```python
from build123d import *

# Parameters (mm, degrees)
F1_DEPTH = 25.4
F2_R     = 4.7625
F3_DEPTH = 12.7


with BuildPart() as f1:
    # F0 (on Right) → F1 (new body, symmetric)
    with BuildSketch(Plane.YZ):
        Polygon((787.4, 9.525), (0, 9.525), (-82.55, 9.525), (-82.55, 0), (-142.875, 0), (-133.35, -9.525), (-33.290768, -9.525), (838.2, -9.525), (838.2, 0), (787.4, 0), align=None)
    extrude(amount=F1_DEPTH, both=True)

    # F2 (on Top) → F3 (cut, symmetric)
    with BuildSketch(Plane.XY):
        with Locations((0, 812.8)):
            Circle(F2_R)
        with Locations((0, 447.675)):
            Circle(F2_R)
    extrude(amount=F3_DEPTH, both=True, mode=Mode.SUBTRACT)


solid = f1.part
```
Design review of the part built by this model. Coordinates are the model's own, in mm. A direction names the side the tool comes from. Give positions to 0.01 mm unless a question says otherwise; leave off trailing zeros. Use a Markdown table: item, result. Add a question column.
(1) Clearance check with flat-ended pins moving along their axes: P1, Ø4, axis at x = 16.5, z = 5, coming from the -Y side; P2, Ø11, axis at x = 0, y = 812.8, coming from the +Z side; P3, Ø11, axis at x = 0, y = 447.675, coming from the -Z side (3 decimals); P4, Ø1, axis at x = 20, z = -6, coming from the -Y side (3 decimals). State where each tip first meets the part, or that it passes through.
(2) Machinability: for faces 1 (the face through (0.4, 807.5, 0)), 2 (the face through (0, -112, 0)), 3 (the face through (-25.4, 341, 0)), which of the approach directions +Z, -Z, +X, -X, +Y, -Y give a long, thin tool a straight path to every point of the face, cutting with its end or side? Answer none if there is none.
(3) Wall thickness on probe 1 along X at (y, z) = (812.8, -5.75); probe 2 along Y at (x, z) = (0, -3) (1 decimal); probe 3 along Y at (x, z) = (0, -3.25) (1 decimal): over which ranges is each line inside the solid? List them lowest first. Write a range as [from, to].
Report:
| question | item | result |
|---|---|---|
| 1 | P1 | stops at y = -82.55 |
| 1 | P2 | stops at z = 0 |
| 1 | P3 | stops at z = -9.525 |
| 1 | P4 | stops at y = -137.375 |
| 2 | face 1 | +Z, +X, -X, +Y |
| 2 | face 2 | +Z, +X, -X, -Y |
| 2 | face 3 | +Z, -Z, -X, +Y, -Y |
| 3 | probe 1 | x = [-25.4, -4.76], [4.76, 25.4] |
| 3 | probe 2 | y = [-139.9, 442.9], [452.4, 808], [817.6, 838.2] |
| 3 | probe 3 | y = [-139.6, 442.9], [452.4, 808], [817.6, 838.2] |
